Can you work these out from the model? Positions are in its coordinate system, mm. A direction names the side the tool comes from. Give positions to 0.01 mm unless a question says otherwise; leave off trailing zeros. Loops run counter-clockwise (first coordinate to the right, second up) from the corner with the lowest first, then second, coordinate; pieces in that order, holes last.
from build123d import *

# Parameters (mm, degrees)
RESSALTO_EXTRUS_O1_DEPTH = 17
ESBO_O3_R                = 5
CORTE_EXTRUS_O2_DEPTH    = 212.497635921
CORTE_EXTRUS_O3_DEPTH    = 20
CHANFRO1_SIZE            = 0.5
ESBO_O5_R                = 6
CORTE_EXTRUS_O4_DEPTH    = 3.5
CORTE_EXTRUS_O4_DRAFT    = -35
FILETE1_R                = 2
ESBO_O6_R                = 2.15
CORTE_EXTRUS_O5_DEPTH    = 212.497636037


with BuildPart() as part:
    # Esbo_o1 → Ressalto-extrus_o1 (new body)
    with BuildSketch(Plane(origin=(0, 0, 0), x_dir=(1, 0, 0), z_dir=(0, 1, 0))):
        with BuildLine():
            Line((0, 17), (194.732173124, 17))
            ThreePointArc((194.732173124, 17), (210, 8.5), (194.732173124, 0))
            Line((194.732173124, 0), (0, 0))
            Line((0, 0), (0, 17))
        make_face()
    extrude(amount=RESSALTO_EXTRUS_O1_DEPTH)

    # Esbo_o3 → Corte-extrus_o2 (cut, through all)
    with BuildSketch(Plane(origin=(0, 17, 0), x_dir=(1, 0, 0), z_dir=(0, 1, 0))):
        with Locations(Location((200, 8.5, 0), (0, 0, 270))):
            Circle(ESBO_O3_R)
    extrude(amount=-CORTE_EXTRUS_O2_DEPTH, mode=Mode.SUBTRACT)

    # Esbo_o4 → Corte-extrus_o3 (cut)
    with BuildSketch(Plane.ZY):
        with BuildLine():
            Line((-7.25, 12.25), (-4.75, 12.25))
            Line((-4.75, 12.25), (-4.75, 9.75))
            ThreePointArc((-4.75, 9.75), (-4.224744871, 8.5), (-4.75, 7.25))
            Line((-4.75, 7.25), (-4.75, 4.75))
            Line((-4.75, 4.75), (-7.25, 4.75))
            ThreePointArc((-7.25, 4.75), (-8.5, 4.224744871), (-9.75, 4.75))
            Line((-9.75, 4.75), (-12.25, 4.75))
            Line((-12.25, 4.75), (-12.25, 7.25))
            ThreePointArc((-12.25, 7.25), (-12.775255129, 8.5), (-12.25, 9.75))
            Line((-12.25, 9.75), (-12.25, 12.25))
            Line((-12.25, 12.25), (-9.75, 12.25))
            ThreePointArc((-9.75, 12.25), (-8.5, 12.775255129), (-7.25, 12.25))
        make_face()
    extrude(amount=-CORTE_EXTRUS_O3_DEPTH, mode=Mode.SUBTRACT)

    # Chanfro1
    chanfro1_edges = [part.edges().sort_by_distance(p)[0] for p in [
        (10, 12.25, -12.25),
        (10, 12.25, -4.75),
        (10, 4.75, -4.75),
        (10, 4.75, -12.25),
    ]]
    chamfer(chanfro1_edges, length=CHANFRO1_SIZE)


with BuildPart() as corte_extrus_o4_tool:
    # Esbo_o5 → Corte-extrus_o4 (with draft: the straight prism first)
    with BuildSketch(Plane.ZY):
        with Locations((-8.5, 8.5)):
            Circle(ESBO_O5_R)
    extrude(amount=-CORTE_EXTRUS_O4_DEPTH)
    # Corte-extrus_o4: the draft: its side faces are tilted about the plane it starts from
    corte_extrus_o4_sides = [corte_extrus_o4_tool.faces().sort_by_distance(p)[0] for p in [
        (1.75, 8.5, -14.5),
    ]]
    draft(corte_extrus_o4_sides, Plane.ZY, CORTE_EXTRUS_O4_DRAFT)


with BuildPart() as part_1:
    add(part.part)

    # Corte-extrus_o4: cut by corte_extrus_o4_tool
    add(corte_extrus_o4_tool.part, mode=Mode.SUBTRACT)

    # Filete1
    filete1_edges = [part_1.edges().sort_by_distance(p)[0] for p in [
        (97.366086562, 17, 0),
        (97.366086562, 0, 0),
        (97.366086562, 0, -17),
        (97.366086562, 17, -17),
    ]]
    fillet(filete1_edges, radius=FILETE1_R)

    # Esbo_o6 → Corte-extrus_o5 (cut, through all)
    with BuildSketch(Plane(origin=(0, 17, 0), x_dir=(1, 0, 0), z_dir=(0, 1, 0))):
        with Locations(Location((8, 8.5, 0), (0, 0, 270))):
            Circle(ESBO_O6_R)
    extrude(amount=-CORTE_EXTRUS_O5_DEPTH, mode=Mode.SUBTRACT)


solid = part_1.part
(1) Thinking about a two-plate mould opening in Y: for faces 1 (the flat face through (106, 0, -9)), 2 (the cylindrical face through (204.957, 8.619, -9.151)), 3 (the flat face through (20, 9, -8)), which applies, pulls with the +Y half, pulls with the -Y half, needs draft (parallel to the pull), parting line crosses it, or undercut?
Returned:
face 1: pulls with the -Y half
face 2: needs draft
face 3: undercut
(2) Which directions (+Z, -Z, +X, -X, +Y, -Y) give clear straight access to the entire face, cutting with the end or side of a thin tool? Please do faces 4 (the flat face through (99, 8, 0)), 5 (the flat face through (96, 8, -17)), 6 (the conical face through (2.416, 6.85, -4.52)).
Returned:
face 4: +Z, -X, +Y, -Y
face 5: -Z, -X, +Y, -Y
face 6: -X
(3) Suppose I cut it at B-B on x = 159. List the corners of the cut face in (y, z) for me.
Returned:
outline: (0, -15) arc R2 ccw to (2, -17) - (15, -17) arc R2 ccw to (17, -15) - (17, -2) arc R2 ccw to (15, 0) - (2, 0) arc R2 ccw to (0, -2) - close
(4) Suppose I cut it at A-A on x = 200. List the corners of the cut face in (y, z) for me, plus the area to 3 significant figures.
Returned:
outline: (0, -18.5) - (17, -18.5) - (17, -13.5) - (0, -13.5) - close; (0, -3.5) - (17, -3.5) - (17, 1.5) - (0, 1.5) - close
area: 170 mm2
(5) Will these pins go through, and if not, where does the flat tip stop? P1, Ø1.6, axis at x = 7, y = 6, coming from the +Z side; P2, Ø3.5, axis at x = 8, z = -8.5, coming from the +Y side; P3, Ø1, axis at x = 33.5, z = -16, coming from the +Y side; P4, Ø1, axis at x = 15, y = 11, coming from the -Z side.
Returned:
P1: stops at z = 0
P2: passes through
P3: stops at y = 16.94
P4: stops at z = -17
(6) Please list where these lines run through material, in increasing order: probe 1 along X at (y, z) = (14.7, -8.5); probe 2 along Z at (x, y) = (8, 2.8); probe 3 along X at (y, z) = (12.75, -7).
Returned:
probe 1: x = 0 to 5.85, 10.15 to 195, 205 to 210
probe 2: z = -17 to -10.65, -6.35 to 0
probe 3: x = 2.13 to 6.46, 9.54 to 195.23, 204.77 to 209.89
